Build history of the part. All positions in model axes, mm. A direction names the side the tool comes from. Give positions to 0.01 mm unless a question says otherwise; leave off trailing zeros. Order: outer loops, then holes, each group sorted by start corner. A loop starts at its lowest first (then second) coordinate and runs counter-clockwise, first axis right, second up. Notation, with made-up numbers: (62.25, -10) - (119.25, -10) arc R10 cw to (119.25, 6) - close; hole circle Ø10 at (8.5, 86). An arc over 180 degrees is marked (long way). Answer in a Markdown table with one row per item.
Solid Edge part; units mm, degrees
sketch "Sketch1" plane through (0, 0, 0) normal (0, -1, 0) x (1, 0, 0)
  line L0 (74.7158, 64.1421) -> (100.5001, 38.3579)
  arc A0 (100.5001, 38.3579) -> (114.6422, 32.5) centre (114.6422, 52.5) ccw
  line L1 (157.6079, 32.5) -> (114.6422, 32.5)
  line L2 (157.6079, 32.5) -> (157.6079, -32.5)
  line L3 (157.6079, -32.5) -> (114.6422, -32.5)
  arc A1 (100.5001, -38.3579) -> (114.6422, -32.5) centre (114.6422, -52.5) cw
  line L4 (74.7158, -64.1421) -> (100.5001, -38.3579)
  arc A2 (60.5737, -70) -> (74.7158, -64.1421) centre (60.5737, -50) ccw
  line L5 (60.5737, -70) -> (-70.3578, -70)
  arc A3 (-84.4999, -64.1421) -> (-70.3578, -70) centre (-70.3578, -50) ccw
  line L6 (-84.4999, -64.1421) -> (-93.2131, -55.4289)
  arc A4 (-100.2842, -52.5) -> (-93.2131, -55.4289) centre (-100.2842, -62.5) cw
  line L7 (-132.3921, -52.5) -> (-100.2842, -52.5)
  line L8 (-132.3921, 52.5) -> (-132.3921, -52.5)
  line L9 (-132.3921, 52.5) -> (-100.2842, 52.5)
  arc A5 (-100.2842, 52.5) -> (-93.2131, 55.4289) centre (-100.2842, 62.5) ccw
  line L10 (-84.4999, 64.1421) -> (-93.2131, 55.4289)
  arc A6 (-84.4999, 64.1421) -> (-70.3578, 70) centre (-70.3578, 50) cw
  line L11 (60.5737, 70) -> (-70.3578, 70)
  arc A7 (60.5737, 70) -> (74.7158, 64.1421) centre (60.5737, 50) cw
extrude "Protrusion1" add sketch "Sketch1" against normal blind 6
sketch "Sketch2" plane through (-2.3921, 6, 0) normal (0, 1, 0) x (-1, 0, 0)
  circle A0 centre (-87.8787, 49.1287) radius 1.5
  circle A1 centre (2.5, 67) radius 1.6
  circle A2 centre (-42.5, 67) radius 1.6
  circle A3 centre (47.5, 67) radius 1.6
  circle A4 centre (87.8787, 54.1287) radius 1.6
  circle A5 centre (-87.8787, -49.1287) radius 1.5
  circle A6 centre (2.5, -67) radius 1.6
  circle A7 centre (-42.5, -67) radius 1.6
  circle A8 centre (47.5, -67) radius 1.6
  circle A9 centre (87.8787, -54.1287) radius 1.6
extrude "ExtrudedCutout_2" cut sketch "Sketch2" along normal mid plane 140
sketch "Sketch3" plane through (-2.3921, 6, 0) normal (0, 1, 0) x (-1, 0, 0)
  circle A0 centre (-147, 60) radius 1.56
  line L0 (-157, -25) -> (-154.9246, -60.4638)
  line L1 (-139.0754, -60.4638) -> (-137, -25)
  line L2 (-157, -25) -> (-137, -25)
  arc A1 (-154.9246, -60.4638) -> (-139.0754, -60.4638) centre (-147, -60) ccw
  circle A2 centre (-147, -60) radius 1.56
  line L3 (-137, 25) -> (-139.0762, 60.4639)
  line L4 (-157, 25) -> (-154.9371, 60.069)
  line L5 (-157, 25) -> (-137, 25)
  arc A3 (-139.0762, 60.4639) -> (-154.9371, 60.069) centre (-147, 60) ccw
extrude "ExtrudedProtrusion_4" add sketch "Sketch3" against normal blind 6
fillet "Round_3" radius 10 4 edges at (154.169, 3, -32.5) (135.0468, 3, -32.5) (154.1667, 3, 32.5) (135.047, 3, 32.5)
1. Which spindle directions (+Z, -Z, +X, -X, +Y, -Y) get a long thin tool onto all of the face, cutting with end or side? Do faces 1 (the face through (136.15, 3.04, -51.32)), 2 (the face through (-117, 3, 52.5)), 3 (the face through (-88.796, 2.958, -59.847)), 4 (the face through (120, 3, 32.5)). Say none if no direction does.
Check result:
| item | result |
|---|---|
| face 1 | -Z, +Y, -Y |
| face 2 | +Z, -X, +Y, -Y |
| face 3 | -Z, -X, +Y, -Y |
| face 4 | +Z, +Y, -Y |
2. Two-plate mould, pull along X, no slides. Class faces 5 (the face through (-96.51, 2.96, 53.24)), 6 (the face through (15, 6, -1)), 7 (the face through (87.43, 2.96, -51.43)): +X half, -X half, draft (parallel to the pull), parting line (faces both ways), or undercut.
Check result:
| item | result |
|---|---|
| face 5 | -X half |
| face 6 | draft |
| face 7 | undercut |
3. Cut at C-C on x = 69. Write the cut outline in (y, z), and give its area (3 significant figures).
Check result:
| item | result |
|---|---|
| outline | (0, -68.14) - (6, -68.14) - (6, 68.14) - (0, 68.14) - close |
| area | 818 mm² |
4. Cut at B-B on y = 4.25. Count the separate pieces of the cut face and the enclosed holes in it, and give its area (3 significant figures).
Check result:
| item | result |
|---|---|
| separate pieces | 1 |
| enclosed holes | 12 |
| area | 34,900 mm² |
5. Cut at A-A on x = 122.5. Write the cut outline in (y, z).
Check result:
| item | result |
|---|---|
| outline | (0, -32.5) - (6, -32.5) - (6, 32.5) - (0, 32.5) - close |
6. Drop flat-ended pins along their axis: P1, Ø2.5, axis at x = 85.49, z = 49.13, coming from the +Y side; P2, Ø1.5, axis at y = 3, z = 56, coming from the +X side; P3, Ø3, axis at x = 122, y = 1.5, coming from the +Z side; P4, Ø5, axis at x = 40.11, z = 67, coming from the +Y side. Give the stop position or say it passes through.
Check result:
| item | result |
|---|---|
| P1 | passes through |
| P2 | stops at x = 152.83 |
| P3 | stops at z = 32.5 |
| P4 | stops at y = 6 |
7. Probe line 1 (Z direction, x = -3.5, y = 3.7); line 2 (X direction, y = 4.75, z = 50); line 3 (Z direction, x = -91, y = 0.25). List the from-to ranges inside material, lowest first.
Check result:
| item | result |
|---|---|
| line 1 | z = -70 to -67.79, -66.21 to 66.21, 67.79 to 70 |
| line 2 | x = -132.39 to 84.27, 86.71 to 88.86, 136.07 to 153.14 |
| line 3 | z = -57.64 to -55.55, -52.7 to 52.7, 55.55 to 57.64 |
